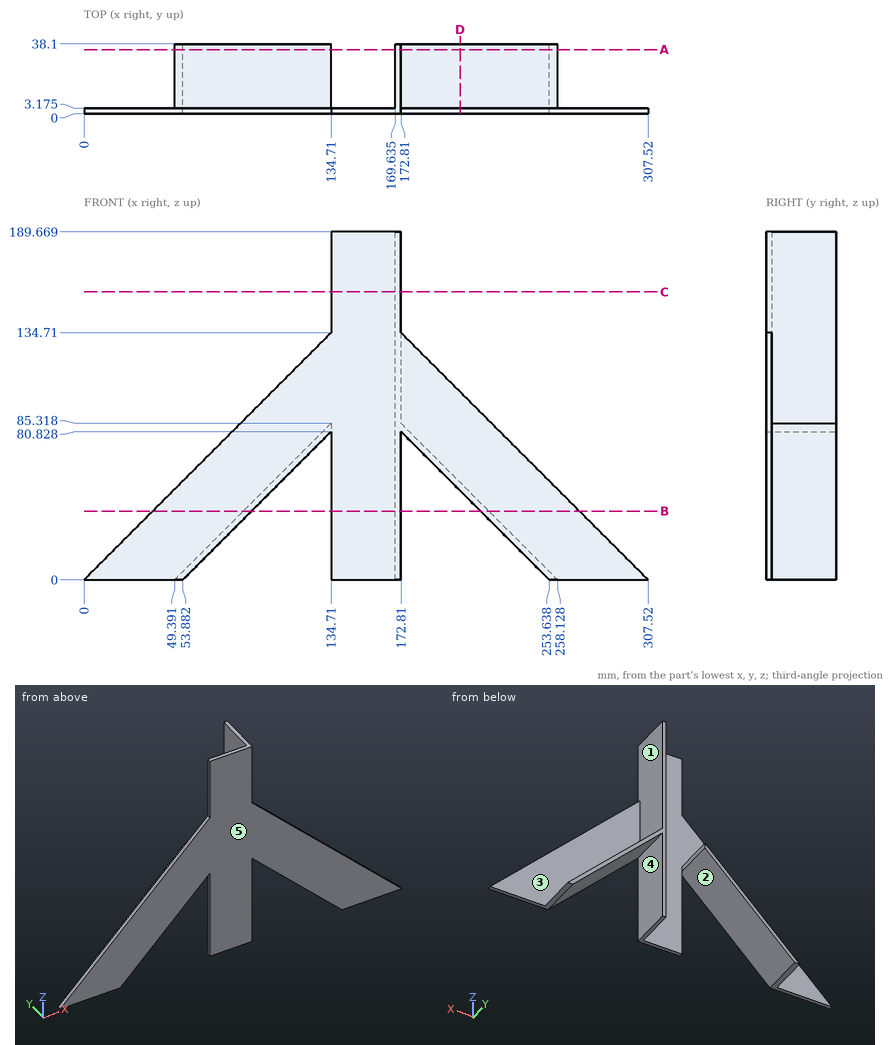
Source: three-view drawing plus pictorial views. Frame: mm from the lowest corner of the part. A direction names the side the tool comes from. Round coordinates to 2 decimals unless told otherwise and drop trailing zeros. Loops run counter-clockwise (first coordinate to the right, second up) from the corner with the lowest first, then second, coordinate; pieces in that order, holes last.
Q1. Ray query, line 1 (X direction, y = 19.5, z = 25) (1 decimal); line 2 (X direction, y = 19.5, z = 37) (1 decimal); line 3 (X direction, y = 20.5, z = 134.5) (1 decimal). Return the intervals inside material, ascending.
Q2. Section D-D, the plane x = 205. Return loops of the section in (y, z) (1 decimal).
Q3. Mould query, pull axis X, two halves, no side actions, for the marked faces 1, 2 and 3. Classes: pulls with the +X half, pulls with the -X half, needs draft (parallel to the pull), parting line crosses it, or undercut.
Q4. Section B-B, the plane z = 37.5. Return loops of the section in (x, y) (1 decimal).
Q5. Section A-A, the plane y = 35. Return loops of the section in (x, z) (1 decimal).
Q6. Section C-C, the plane z = 157. Return loops of the section in (x, y) (1 decimal).
Q7. First-contact query: P1, Ø2.5, axis at y = 1.5, z = 37, coming from the -X side; P2, Ø1.5, axis at x = 201, y = 22, coming from the -Z side; P3, Ø3.5, axis at y = 13, z = 83, coming from the +X side. Flat tips, straight axial feed; report the tip coordinate or a pass-through.
Q8. Access query for the marked faces 4 and 5. Directions: +Z, -Z, +X, -X, +Y, -Y. A direction counts if a zero-diameter tool reaches every point of the face in a straight line with its end or side. Return the directions, or none.
Solutions:
1. line 1: x = 74.4 to 78.9, 169.6 to 172.8, 228.6 to 233.1
1. line 2: x = 86.4 to 90.9, 169.6 to 172.8, 216.6 to 221.1
1. line 3: x = 169.6 to 172.8
2. outline: (0, 48.6) - (38.1, 48.6) - (38.1, 53.1) - (3.2, 53.1) - (3.2, 102.5) - (0, 102.5) - close
3. face 1: pulls with the +X half
3. face 2: undercut
3. face 3: needs draft
4. outline: (37.5, 0) - (91.4, 0) - (91.4, 38.1) - (86.9, 38.1) - (86.9, 3.2) - (37.5, 3.2) - close; (134.7, 0) - (172.8, 0) - (172.8, 38.1) - (169.6, 38.1) - (169.6, 3.2) - (134.7, 3.2) - close; (216.1, 0) - (270, 0) - (270, 3.2) - (220.6, 3.2) - (220.6, 38.1) - (216.1, 38.1) - close
5. outline: (49.4, 0) - (53.9, 0) - (134.7, 80.8) - (134.7, 85.3) - close; (169.6, 0) - (172.8, 0) - (172.8, 80.8) - (253.6, 0) - (258.1, 0) - (172.8, 85.3) - (172.8, 189.7) - (169.6, 189.7) - close
6. outline: (134.7, 0) - (172.8, 0) - (172.8, 38.1) - (169.6, 38.1) - (169.6, 3.2) - (134.7, 3.2) - close
7. P1: stops at x = 35.75
7. P2: stops at z = 51.89
7. P3: stops at x = 176.88
8. face 4: -Z, +Y, -Y
8. face 5: +Z, -Z, +X, -X, -Y
